Source: CAD feature listing. Evaluate the final solid. Frame: model axes, mm. A direction names the side the tool comes from. Round coordinates to 2 decimals unless told otherwise and drop trailing zeros. Loops run counter-clockwise (first coordinate to the right, second up) from the corner with the lowest first, then second, coordinate; pieces in that order, holes last. Notation, with made-up numbers: (14.25, -24) -> (57.25, -24) arc R29 ccw to (57.25, -4) -> close; hole circle Ø5 at (-11.75, 24.5). An arc over 180 degrees is marked (long way). Put each result on its own line as item: value. Start each with the question number.
1. Cut plane C-C (x = 5). Return the cut outline in (y, z) (3 decimals).
2. Draft query along X for faces 3 (the flat face through (-53.975, 0, -9)), 4 (the flat face through (-4, 4.8, -9.4)), 5 (the flat face through (-1, 0, -19.05)). Return one class per face: pulls with the +X half, pulls with the -X half, needs draft (parallel to the pull), parting line crosses it, or undercut.
3. Cut plane B-B (z = -13.5). Return the cut outline in (x, y) (1 decimal).
4. Material intervals for L1, parallel to X at y = 1.75, z = -14.75 (3 decimals); L2, parallel to X at y = 7.5, z = -18 (3 decimals); L3, parallel to Y at x = -7, z = -11 (3 decimals), sorted ascending.
5. Set-up query: faces 1 (the flat face through (3.913, 4.696, -9.392)), 2 (the flat face through (53.975, 0, -9)). Return all of +Z, -Z, +X, -X, +Y, -Y with unobstructed straight access to the full face (end or side cutting, diameter ignored); none if empty.
6. Cut plane A-A (y = 4.5). Return the cut outline in (x, z) (3 decimals).
```python
from build123d import *

# Parameters (mm, degrees)
F0_W     = 107.95
F0_H     = 19.05
F1_DEPTH = 19.05
F3_DEPTH = 25.4
F5_D     = 1.5875


with BuildPart() as f1:
    # F0 (on Top) → F1 (new body)
    with BuildSketch(Plane.XY):
        Rectangle(F0_W, F0_H)
    extrude(amount=-F1_DEPTH)

    # F2 (on face) → F3 (cut)
    with BuildSketch(Plane.XY):
        Polygon((-7.9375, 9.525), (0, 0), (7.9375, 9.525), align=None)
    extrude(amount=-F3_DEPTH, mode=Mode.SUBTRACT)

    # F5 (through all)
    with Locations(Plane.XY):
        with Locations((-52.3875, 0)):
            Hole(F5_D / 2)


solid = f1.part
```
Solution:
1. outline: (-9.525, -19.05) -> (6, -19.05) -> (6, 0) -> (-9.525, 0) -> close
2. face 3: pulls with the -X half
2. face 4: undercut
2. face 5: needs draft
3. outline: (-54, -9.5) -> (54, -9.5) -> (54, 9.5) -> (7.9, 9.5) -> (0, 0) -> (-7.9, 9.5) -> (-54, 9.5) -> close; hole circle Ø1.6 at (-52.4, 0)
4. L1: x = -53.975 to -1.458, 1.458 to 53.975
4. L2: x = -53.975 to -6.25, 6.25 to 53.975
4. L3: y = -9.525 to 8.4
5. face 1: +Z, -Z, +Y
5. face 2: +Z, -Z, +X, +Y, -Y
6. outline: (-53.975, -19.05) -> (-3.75, -19.05) -> (-3.75, 0) -> (-53.975, 0) -> close; (3.75, -19.05) -> (53.975, -19.05) -> (53.975, 0) -> (3.75, 0) -> close
